The listing builds one solid part. Answer for the finished solid, in the listing's coordinates (mm). Face numbers are marked on the shaded views. A direction names the side the tool comes from. Give positions to 0.01 mm unless a question says otherwise; leave off trailing zeros. Write each loop counter-clockwise with the first axis right and the second up, starting at its lowest first coordinate (ties: lowest second). Pieces come first, ordered by that corner, then holes.
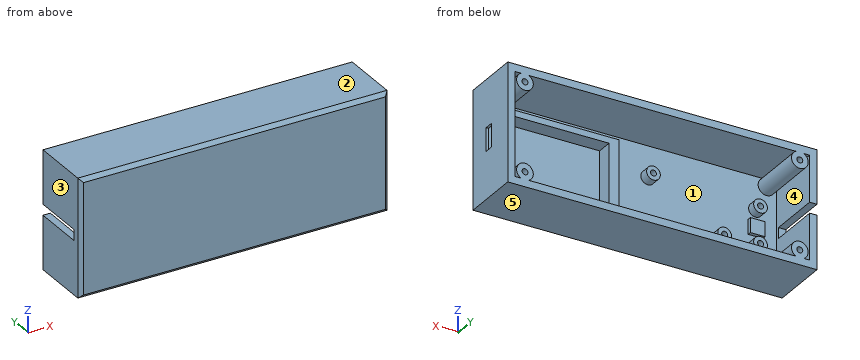
```python
from build123d import *

# Parameters (mm, degrees)
SKETCH1_W           = 126
SKETCH1_H           = 48
BOSS_EXTRUDE1_DEPTH = 25.5
CHAMFER1_SIZE       = 1.5
SKETCH2_W           = 120
SKETCH2_H           = 42
CUT_EXTRUDE1_DEPTH  = 23
SKETCH3_R           = 3.4
BOSS_EXTRUDE2_DEPTH = 25.5
SKETCH4_R           = 1.2
CUT_EXTRUDE2_DEPTH  = 13
SKETCH5_R           = 2.8
BOSS_EXTRUDE3_DEPTH = 6.5
SKETCH6_R           = 1.2
CUT_EXTRUDE3_DEPTH  = 5
SKETCH7_R           = 2.8
BOSS_EXTRUDE4_DEPTH = 6
SKETCH8_W           = 6
SKETCH8_H           = 6
BOSS_EXTRUDE5_DEPTH = 4
SKETCH9_R           = 1.2
CUT_EXTRUDE4_DEPTH  = 5
SKETCH10_W          = 5
SKETCH10_H          = 4.4
CUT_EXTRUDE5_DEPTH  = 21.5
SKETCH11_W          = 52
SKETCH11_H          = 32
SKETCH11_W_2        = 46
SKETCH11_H_2        = 27
BOSS_EXTRUDE6_DEPTH = 9
SKETCH12_W          = 28.4
SKETCH12_H          = 7
CUT_EXTRUDE7_DEPTH  = 2
SKETCH13_W          = 9.5
SKETCH13_H          = 3.8
CUT_EXTRUDE8_DEPTH  = 2


with BuildPart() as part:
    # Sketch1 → Boss-Extrude1 (new body)
    with BuildSketch(Plane(origin=(0, 0, 0), x_dir=(1, 0, 0), z_dir=(0, 1, 0))):
        Rectangle(SKETCH1_W, SKETCH1_H)
    extrude(amount=BOSS_EXTRUDE1_DEPTH)

    # Chamfer1
    chamfer1_edges = [part.edges().sort_by_distance(p)[0] for p in [
        (0, 0, -24),
        (63, 0, 0),
        (0, 0, 24),
        (-63, 0, 0),
    ]]
    chamfer(chamfer1_edges, length=CHAMFER1_SIZE)

    # Sketch2 → Cut-Extrude1 (cut)
    with BuildSketch(Plane(origin=(0, 25.5, 0), x_dir=(1, 0, 0), z_dir=(0, 1, 0))):
        Rectangle(SKETCH2_W, SKETCH2_H)
    extrude(amount=-CUT_EXTRUDE1_DEPTH, mode=Mode.SUBTRACT)

    # Sketch3 → Boss-Extrude2 (add)
    with BuildSketch(Plane(origin=(0, 0, 0), x_dir=(1, 0, 0), z_dir=(0, 1, 0))):
        with Locations((-56, 18)):
            Circle(SKETCH3_R)
        with Locations((-56, -18)):
            Circle(SKETCH3_R)
        with Locations((56, 18)):
            Circle(SKETCH3_R)
        with Locations((56, -18)):
            Circle(SKETCH3_R)
    extrude(amount=BOSS_EXTRUDE2_DEPTH)

    # Sketch4 → Cut-Extrude2 (cut)
    with BuildSketch(Plane(origin=(0, 25.5, 0), x_dir=(1, 0, 0), z_dir=(0, 1, 0))):
        with Locations(Location((-56, 18, 0), (0, 0, 270))):
            Circle(SKETCH4_R)
        with Locations(Location((-56, -18, 0), (0, 0, 270))):
            Circle(SKETCH4_R)
        with Locations(Location((56, 18, 0), (0, 0, 270))):
            Circle(SKETCH4_R)
        with Locations(Location((56, -18, 0), (0, 0, 270))):
            Circle(SKETCH4_R)
    extrude(amount=-CUT_EXTRUDE2_DEPTH, mode=Mode.SUBTRACT)

    # Sketch5 → Boss-Extrude3 (add)
    with BuildSketch(Plane(origin=(0, 0, 0), x_dir=(1, 0, 0), z_dir=(0, 1, 0))):
        with Locations(Location((-36.59, 8.21, 0), (0, 0, 90))):
            Circle(SKETCH5_R)
        with Locations(Location((-7.59, -8.21, 0), (0, 0, 90))):
            Circle(SKETCH5_R)
    extrude(amount=BOSS_EXTRUDE3_DEPTH)

    # Sketch6 → Cut-Extrude3 (cut)
    with BuildSketch(Plane(origin=(0, 6.5, 0), x_dir=(1, 0, 0), z_dir=(0, 1, 0))):
        with Locations(Location((-36.59, 8.21, 0), (0, 0, 270))):
            Circle(SKETCH6_R)
        with Locations(Location((-7.59, -8.21, 0), (0, 0, 270))):
            Circle(SKETCH6_R)
    extrude(amount=-CUT_EXTRUDE3_DEPTH, mode=Mode.SUBTRACT)

    # Sketch7 → Boss-Extrude4 (add)
    with BuildSketch(Plane(origin=(0, 0, 0), x_dir=(1, 0, 0), z_dir=(0, 1, 0))):
        with Locations(Location((-51.5, 7.5, 0), (0, 0, 90))):
            Circle(SKETCH7_R)
        with Locations(Location((-51.5, -7.5, 0), (0, 0, 90))):
            Circle(SKETCH7_R)
    extrude(amount=BOSS_EXTRUDE4_DEPTH)

    # Sketch8 → Boss-Extrude5 (add)
    with BuildSketch(Plane(origin=(0, 0, 0), x_dir=(1, 0, 0), z_dir=(0, 1, 0))):
        with Locations((-51.5, 0)):
            Rectangle(SKETCH8_W, SKETCH8_H)
    extrude(amount=BOSS_EXTRUDE5_DEPTH)

    # Sketch9 → Cut-Extrude4 (cut)
    with BuildSketch(Plane(origin=(0, 6, 0), x_dir=(1, 0, 0), z_dir=(0, 1, 0))):
        with Locations(Location((-51.5, 7.5, 0), (0, 0, 270))):
            Circle(SKETCH9_R)
        with Locations(Location((-51.5, -7.5, 0), (0, 0, 270))):
            Circle(SKETCH9_R)
    extrude(amount=-CUT_EXTRUDE4_DEPTH, mode=Mode.SUBTRACT)

    # Sketch10 → Cut-Extrude5 (cut)
    with BuildSketch(Plane(origin=(0, 25.5, 0), x_dir=(1, 0, 0), z_dir=(0, 1, 0))):
        with Locations((-61.5, 0)):
            Rectangle(SKETCH10_W, SKETCH10_H)
    extrude(amount=-CUT_EXTRUDE5_DEPTH, mode=Mode.SUBTRACT)

    # Sketch11 → Boss-Extrude6 (add)
    with BuildSketch(Plane(origin=(0, 0, 0), x_dir=(1, 0, 0), z_dir=(0, 1, 0))):
        with Locations((34, 0)):
            Rectangle(SKETCH11_W, SKETCH11_H)
        with Locations((35, 0)):
            Rectangle(SKETCH11_W_2, SKETCH11_H_2, mode=Mode.SUBTRACT)
    extrude(amount=BOSS_EXTRUDE6_DEPTH)

    # Sketch12 → Cut-Extrude7 (cut)
    with BuildSketch(Plane(origin=(60, 0, 0), x_dir=(0, 0, -1), z_dir=(1, 0, 0))):
        with Locations((0, 12.5)):
            Rectangle(SKETCH12_W, SKETCH12_H)
    extrude(amount=CUT_EXTRUDE7_DEPTH, mode=Mode.SUBTRACT)

    # Sketch13 → Cut-Extrude8 (cut)
    with BuildSketch(Plane(origin=(63, 0, 0), x_dir=(0, 0, -1), z_dir=(1, 0, 0))):
        with Locations((0, 12.4)):
            Rectangle(SKETCH13_W, SKETCH13_H)
    extrude(amount=-CUT_EXTRUDE8_DEPTH, mode=Mode.SUBTRACT)


solid = part.part
```
Item 1: A cutting plane is placed at A-A, the plane y = 21.5. Give the vertices of the cut face in (x, z), plus the area to 3 significant figures.
Conclusion:
outline: (-63, -24) - (63, -24) - (63, 24) - (-63, 24) - (-63, 2.2) - (-60, 2.2) - (-60, 21) - (-57.6, 21) arc R3.4 ccw (long way) to (-54.4, 21) - (54.4, 21) arc R3.4 ccw (long way) to (57.6, 21) - (60, 21) - (60, -21) - (57.6, -21) arc R3.4 ccw (long way) to (54.4, -21) - (-54.4, -21) arc R3.4 ccw (long way) to (-57.6, -21) - (-60, -21) - (-60, -2.2) - (-63, -2.2) - close; hole circle Ø2.4 at (-56, -18); hole circle Ø2.4 at (-56, 18); hole circle Ø2.4 at (56, -18); hole circle Ø2.4 at (56, 18)
area: 1,120 mm2
Item 2: A cutting plane is placed at C-C, the plane z = -18. Give the vertices of the cut face in (x, y), plus the area to 3 significant figures.
Conclusion:
outline: (-63, 1.5) - (-61.5, 0) - (61.5, 0) - (63, 1.5) - (63, 25.5) - (60, 25.5) - (60, 2.5) - (59.4, 2.5) - (59.4, 25.5) - (57.2, 25.5) - (57.2, 12.5) - (54.8, 12.5) - (54.8, 25.5) - (52.6, 25.5) - (52.6, 2.5) - (-52.6, 2.5) - (-52.6, 25.5) - (-54.8, 25.5) - (-54.8, 12.5) - (-57.2, 12.5) - (-57.2, 25.5) - (-59.4, 25.5) - (-59.4, 2.5) - (-60, 2.5) - (-60, 25.5) - (-63, 25.5) - close
area: 701 mm2
Item 3: A cutting plane is placed at D-D, the plane x = 56. Give the vertices of the cut face in (y, z).
Conclusion:
outline: (0, -22.5) - (1.5, -24) - (25.5, -24) - (25.5, -19.2) - (12.5, -19.2) - (12.5, -16.8) - (25.5, -16.8) - (25.5, -14.6) - (9, -14.6) - (9, -13.5) - (2.5, -13.5) - (2.5, 13.5) - (9, 13.5) - (9, 14.6) - (25.5, 14.6) - (25.5, 16.8) - (12.5, 16.8) - (12.5, 19.2) - (25.5, 19.2) - (25.5, 24) - (1.5, 24) - (0, 22.5) - close
Item 4: Which of the six approach directions +Z, -Z, +X, -X, +Y, -Y give full straight-line access (tool end or side, diameter ignored) to the marked faces 4 and 5?
Conclusion:
face 4: +Y
face 5: -Z, +X, -X, +Y, -Y
Item 5: Each of these flat-tipped pins is pushed along its axis until it touches: P1, Ø4, axis at x = 48, z = -8.5, coming from the +Y side; P2, Ø1.7, axis at x = -51.5, z = 6.5, coming from the +Y side; P3, Ø1.8, axis at x = -52, z = 0, coming from the +Y side. Where does it stop, or does it pass through?
Conclusion:
P1: stops at y = 2.5
P2: stops at y = 6
P3: stops at y = 4
Item 6: Determine the mould class of the marked faces 1, 2 and 3 for opening direction X: pulls with the +X half, pulls with the -X half, needs draft (parallel to the pull), parting line crosses it, or undercut.
Conclusion:
face 1: undercut
face 2: needs draft
face 3: pulls with the -X half
Item 7: Consider probe 1 along Z at (x, y) = (15, 8.75); probe 2 along X at (y, z) = (7.5, 9); probe 3 along Z at (x, y) = (-17.5, 22). Determine where each line is inside the solid, lowest interval first.
Conclusion:
probe 1: z = -24 to -21, -16 to -13.5, 13.5 to 16, 21 to 24
probe 2: x = -63 to -60, 8 to 12, 58 to 63
probe 3: z = -24 to -21, 21 to 24
